Build history of the part. All positions in model axes, mm. Face numbers are marked on the shaded views. A direction names the side the tool comes from. Round coordinates to 2 decimals unless told otherwise and drop trailing zeros. Loops run counter-clockwise (first coordinate to the right, second up) from the corner with the lowest first, then second, coordinate; pieces in that order, holes last.
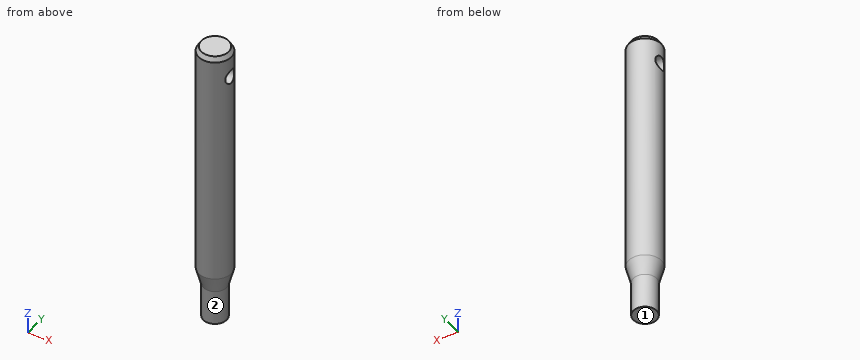
from build123d import *

# Parameters (mm, degrees)
F0_R          = 7
F1_DEPTH      = 62.5
F2_R          = 3
F3_DEPTH      = 7.001
F3_DEPTH_BACK = 7.001
F6_SIZE2      = 1.1547005384
F6_SIZE       = 2


with BuildPart() as f1:
    # F0 (on Top) → F1 (new body, symmetric)
    with BuildSketch(Plane.XY):
        Circle(F0_R)
    extrude(amount=F1_DEPTH, both=True)

    # F2 (on Right) → F3 (cut, two sides)
    with BuildSketch(Plane.YZ) as f3_sk:
        with Locations((0, 51.5)):
            Circle(F2_R)
    extrude(amount=-F3_DEPTH, mode=Mode.SUBTRACT)
    extrude(f3_sk.sketch, amount=F3_DEPTH_BACK, mode=Mode.SUBTRACT)

    # F4 (on Right) → F5 (revolve, cut)
    with BuildSketch(Plane.YZ):
        Polygon((-5, -47.5), (-7, -40.0358983849), (-7, -62.5), (-5, -62.5), align=None)
    revolve(axis=Axis((0, 0, -51.2679491924), (0, 0, 1)), mode=Mode.SUBTRACT)

    # F6
    f6_edges = [f1.edges().sort_by_distance(p)[0] for p in [
        (-7, 0, 62.5),
    ]]
    f6_side = f1.faces().sort_by_distance((-7, 0, 11.232051))[0]
    chamfer(f6_edges, length=F6_SIZE, length2=F6_SIZE2, reference=f6_side)


solid = f1.part
(1) Pin check, flat tips, straight feed: P1, Ø3, axis at y = 5.5, z = 8, coming from the -X side; P2, Ø1, axis at y = -3.5, z = 6, coming from the +X side; P3, Ø2, axis at x = -4, z = -19.5, coming from the +Y side. Stop position of each tip, or through.
Responses:
P1: stops at x = -5.74
P2: stops at x = 6.32
P3: stops at y = 6.32
(2) Which spindle directions (+Z, -Z, +X, -X, +Y, -Y) get a long thin tool onto all of the face, cutting with end or side? Do the marked faces 1 and 2. Say none if no direction does.
Responses:
face 1: -Z, +X, -X, +Y, -Y
face 2: -Z
(3) Slice it at C-C on z = 51.5. List the corners of the cut face in (x, y), plus the area to 3 significant figures.
Responses:
outline: (-6.32, -3) arc R7 ccw to (6.32, -3) - close; (-6.32, 3) - (6.32, 3) arc R7 ccw to start
area: 72.6 mm2
(4) Slice it at A-A on y = 0. List the corners of the cut face in (x, z).
Responses:
outline: (-7, -40.04) - (-5, -47.5) - (-5, -62.5) - (5, -62.5) - (5, -47.5) - (7, -40.04) - (7, 48.5) - (-7, 48.5) - close; (-7, 54.5) - (7, 54.5) - (7, 60.5) - (5.85, 62.5) - (-5.85, 62.5) - (-7, 60.5) - close
(5) Probe line 1 (Z direction, x = -2, y = 0); line 2 (X direction, y = 0.25, z = -48); line 3 (Z direction, x = -2, y = 1). List the from-to ranges inside material, lowest first.
Responses:
line 1: z = -62.5 to 48.5, 54.5 to 62.5
line 2: x = -4.99 to 4.99
line 3: z = -62.5 to 48.67, 54.33 to 62.5
(6) Slice it at B-B on z = 12. List the corners of the cut face in (x, y).
Responses:
outline: circle Ø14 at (0, 0)
